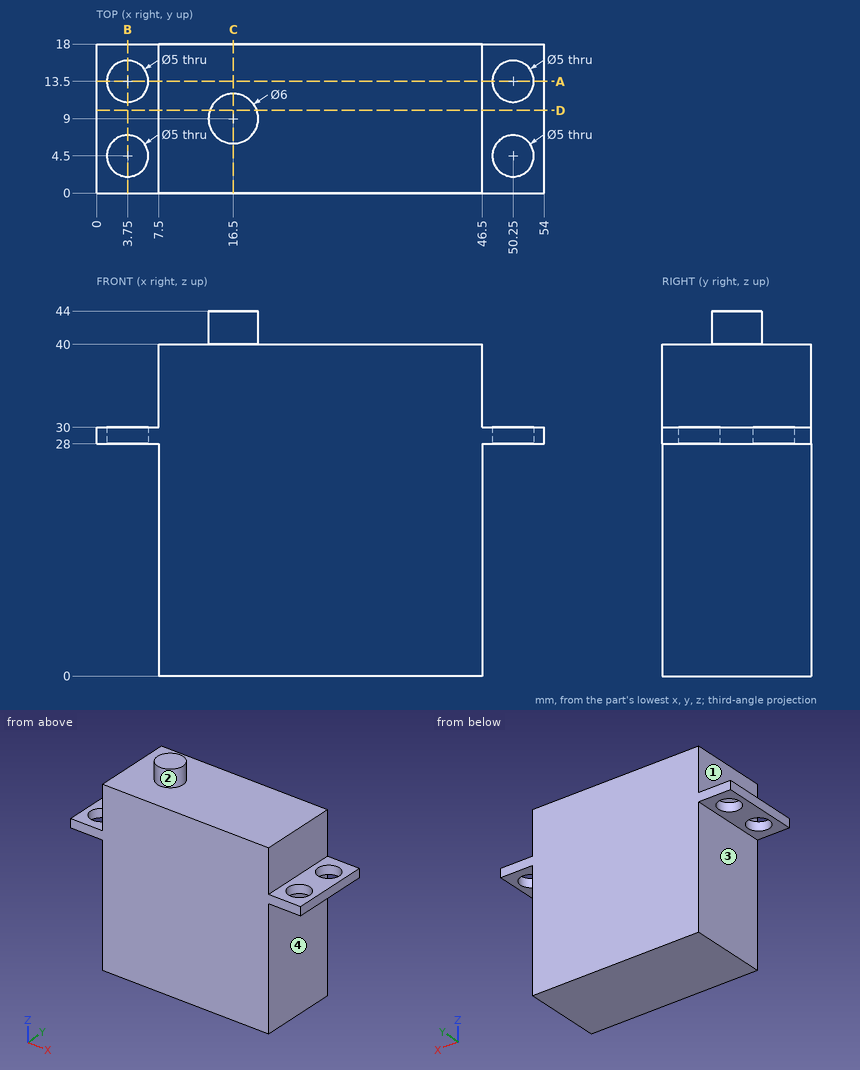
For this review, use the dimensioned drawing (mm, ordinates from the lowest corner) and the shaded views. A direction names the side the tool comes from. Coordinates: 2 decimals unless noted, no trailing zeros. Loops run counter-clockwise (first coordinate to the right, second up) from the corner with the lowest first, then second, coordinate; pieces in that order, holes last. Notation, with made-up numbers: (40, 88.5) - (61, 88.5) arc R27 cw to (61, 117.5) - close; hole circle Ø5 at (32.5, 64). An arc over 180 degrees is marked (long way). Use CSV: the item, a comma, the result in double quotes. Start each with the question number.
1) For pin 1 Ø4 at (x, z) = (48, 18.5) entering from -Y; pin 2 Ø1.5 at (y, z) = (3, 4.5) entering from -X; pin 3 Ø6 at (x, y) = (50.25, 4.5) entering from -Z; pin 4 Ø3 at (x, y) = (15, 2) entering from +Z, all flat-tipped, find the tip position at first contact; note any pin that passes through.
2) Consider section A-A on y = 13.5. Write out the cut boundary in (x, z), then the cut area to 3 significant figures.
3) Consider section D-D on y = 10. Write out the cut boundary in (x, z).
4) Tool access review of the marked faces 1, 2, 3 and 4: name each direction out of +Z, -Z, +X, -X, +Y, -Y from which nothing blocks a thin tool from reaching the whole face with its end or side.
5) Wall thickness on L1, parallel to Y at x = 3.75, z = 29.25; L2, parallel to X at y = 15, z = 29; L3, parallel to Z at x = 32, y = 15.5: over which ranges is each line inside the solid? List them lowest first. Write a range as from..to.
6) Consider section B-B on x = 3.75. Write out the cut boundary in (y, z), then the cut area to 3 significant figures.
7) Consider section C-C on x = 16.5. Write out the cut boundary in (y, z), then the cut area to 3 significant figures.
Geometry says:
1,pin 1,"y = 0"
1,pin 2,"x = 7.5"
1,pin 3,"z = 28"
1,pin 4,"z = 40"
2,outline,"(0, 28) - (1.25, 28) - (1.25, 30) - (0, 30) - close; (6.25, 28) - (7.5, 28) - (7.5, 0) - (46.5, 0) - (46.5, 28) - (47.75, 28) - (47.75, 30) - (46.5, 30) - (46.5, 40) - (7.5, 40) - (7.5, 30) - (6.25, 30) - close; (52.75, 28) - (54, 28) - (54, 30) - (52.75, 30) - close"
2,area,"1,570 mm^2"
3,outline,"(0, 28) - (7.5, 28) - (7.5, 0) - (46.5, 0) - (46.5, 28) - (54, 28) - (54, 30) - (46.5, 30) - (46.5, 40) - (19.33, 40) - (19.33, 44) - (13.67, 44) - (13.67, 40) - (7.5, 40) - (7.5, 30) - (0, 30) - close"
4,face 1,"+Z, -X, +Y, -Y"
4,face 2,"+Z"
4,face 3,"-Z, -X, +Y, -Y"
4,face 4,"-Z, +X, +Y, -Y"
5,L1,"0..2, 7..11, 16..18"
5,L2,"0..1.75, 5.75..48.25, 52.25..54"
5,L3,"0..40"
6,outline,"(0, 28) - (2, 28) - (2, 30) - (0, 30) - close; (7, 28) - (11, 28) - (11, 30) - (7, 30) - close; (16, 28) - (18, 28) - (18, 30) - (16, 30) - close"
6,area,"16.0 mm^2"
7,outline,"(0, 0) - (18, 0) - (18, 40) - (12, 40) - (12, 44) - (6, 44) - (6, 40) - (0, 40) - close"
7,area,"744 mm^2"
